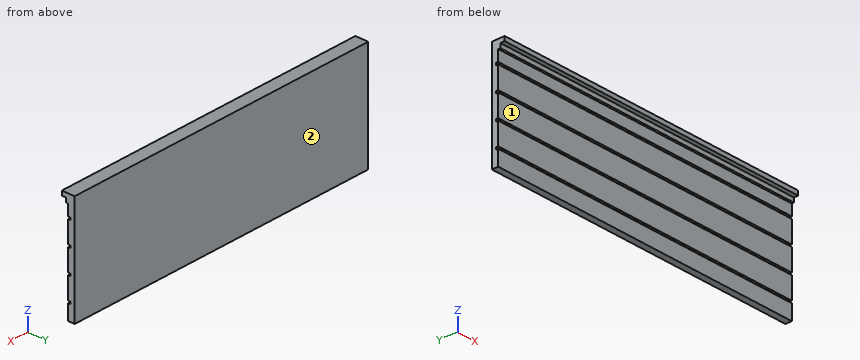
from build123d import *

# Parameters (mm, degrees)
SKETCH1_W           = 149
SKETCH1_H           = 50
BOSS_EXTRUDE1_DEPTH = 3
SKETCH2_W           = 149
SKETCH2_H           = 1
CUT_EXTRUDE1_DEPTH  = 1
SKETCH3_W           = 149
SKETCH3_H           = 4
BOSS_EXTRUDE2_DEPTH = 1
SKETCH4_W           = 149
SKETCH4_H           = 2
BOSS_EXTRUDE3_DEPTH = 2


with BuildPart() as part:
    # Sketch1 → Boss-Extrude1 (new body)
    with BuildSketch(Plane(origin=(0, 0, 0), x_dir=(1, 0, 0), z_dir=(0, 1, 0))):
        Rectangle(SKETCH1_W, SKETCH1_H)
    extrude(amount=BOSS_EXTRUDE1_DEPTH)

    # Sketch2 → Cut-Extrude1 (cut)
    with BuildSketch(Plane.XZ):
        with Locations((0, -17.5)):
            Rectangle(SKETCH2_W, SKETCH2_H)
        with Locations((0, -6.5)):
            Rectangle(SKETCH2_W, SKETCH2_H)
        with Locations((0, 4.5)):
            Rectangle(SKETCH2_W, SKETCH2_H)
        with Locations((0, 15.5)):
            Rectangle(SKETCH2_W, SKETCH2_H)
    extrude(amount=-CUT_EXTRUDE1_DEPTH, mode=Mode.SUBTRACT)

    # Sketch3 → Boss-Extrude2 (add)
    with BuildSketch(Plane.XZ):
        with Locations((0, 23)):
            Rectangle(SKETCH3_W, SKETCH3_H)
    extrude(amount=BOSS_EXTRUDE2_DEPTH)

    # Sketch4 → Boss-Extrude3 (add)
    with BuildSketch(Plane.XZ.offset(1)):
        with Locations((0, 24)):
            Rectangle(SKETCH4_W, SKETCH4_H)
    extrude(amount=BOSS_EXTRUDE3_DEPTH)


solid = part.part
Check sheet for the modelled part. Datum: model origin and axes. Units: mm. Face numbers are marked on the shaded views. A direction names the side the tool comes from. Give positions to 0.01 mm unless a question says otherwise; leave off trailing zeros. Order: outer loops, then holes, each group sorted by start corner. A loop starts at its lowest first (then second) coordinate and runs counter-clockwise, first axis right, second up. Notation, with made-up numbers: M 69,53.25 L 73,53.25 A30 ccw 73,78.25 Z; hole C 73,27.25 d4. An arc over 180 degrees is marked long. Answer as CSV lines item,"result". Start each with the question number.
Item 1: Thickness scan on line 1 (Z direction, x = -11.5, y = 0.65); line 2 (Y direction, x = -14, z = 22); line 3 (Z direction, x = 3.5, y = -1.65). Record the ranges inside material, lowest first. Write a range as [from, to].
Item 2: Tool access check on the marked faces 1 and 2. Record the directions out of +Z, -Z, +X, -X, +Y, -Y that give a thin tool (end or side, any length) a straight path to the whole face; none if there is none.
Item 3: Cross-section at A-A on x = -2. Enter the section's corners in (y, z), plus the area to 3 significant figures.
Item 4: Cross-section at B-B on z = -21. Enter the section's corners in (x, y).
Item 5: Cross-section at C-C on y = -2.1. Enter the section's corners in (x, z).
Item 6: Gauge pin test, flat ends, axial feed: P1, Ø0.6, axis at x = 25.5, z = 22.5, coming from the -Y side; P2, Ø11, axis at x = -29, z = 1.5, coming from the -Y side; P3, Ø0.5, axis at x = 29.5, y = -0.5, coming from the -Z side. Record the tip position at first contact, or that the pin passes through.
Established:
1,line 1,"z = [-25, -18], [-17, -7], [-6, 4], [5, 15], [16, 25]"
1,line 2,"y = [-1, 3]"
1,line 3,"z = [23, 25]"
2,face 1,"-Z, +X, -X, -Y"
2,face 2,"+Z, -Z, +X, -X, +Y"
3,outline,"M -3,23 L -1,23 L -1,21 L 0,21 L 0,16 L 1,16 L 1,15 L 0,15 L 0,5 L 1,5 L 1,4 L 0,4 L 0,-6 L 1,-6 L 1,-7 L 0,-7 L 0,-17 L 1,-17 L 1,-18 L 0,-18 L 0,-25 L 3,-25 L 3,25 L -3,25 Z"
3,area,"154 mm^2"
4,outline,"M -74.5,0 L 74.5,0 L 74.5,3 L -74.5,3 Z"
5,outline,"M -74.5,23 L 74.5,23 L 74.5,25 L -74.5,25 Z"
6,P1,"stops at y = -1"
6,P2,"stops at y = 0"
6,P3,"stops at z = 21"
